Work out the finished part from the listing and answer in its coordinate system (mm). Face numbers are marked on the shaded views. Coordinates: 2 decimals unless noted, no trailing zeros. Write each loop counter-clockwise with the first axis right and the second up, starting at its lowest first coordinate (ties: lowest second). Pieces come first, ordered by that corner, then holes. Notation, with made-up numbers: M 52,4 L 71,4 A36 cw 71,39 Z; hole C 8.25,53.5 d11. An arc over 180 degrees is marked long. Use CSV: the item, a comma, the result in double quotes.
from build123d import *


with BuildPart() as part:
    # Sketch1 → Revolve1 (revolve)
    with BuildSketch(Plane.XZ):
        with BuildLine():
            Line((14.2875, 0.508), (14.2875, 5.89534))
            Line((14.2875, 5.89534), (13.97, 5.89534))
            Line((13.97, 5.89534), (13.97, 6.40334))
            Line((13.97, 6.40334), (15.4305, 6.40334))
            Line((15.4305, 6.40334), (15.5575, 6.53034))
            Line((15.5575, 6.53034), (15.5575, 7.80034))
            Line((15.5575, 7.80034), (15.4305, 7.92734))
            Line((15.4305, 7.92734), (6.35, 7.92734))
            Line((6.35, 7.92734), (6.35, 0))
            Line((6.35, 0), (13.7795, 0))
            ThreePointArc((13.7795, 0), (14.138710245, 0.148789755), (14.2875, 0.508))
        make_face()
    revolve(axis=Axis((0, 0, 7.92734), (0, 0, -1)))


solid = part.part
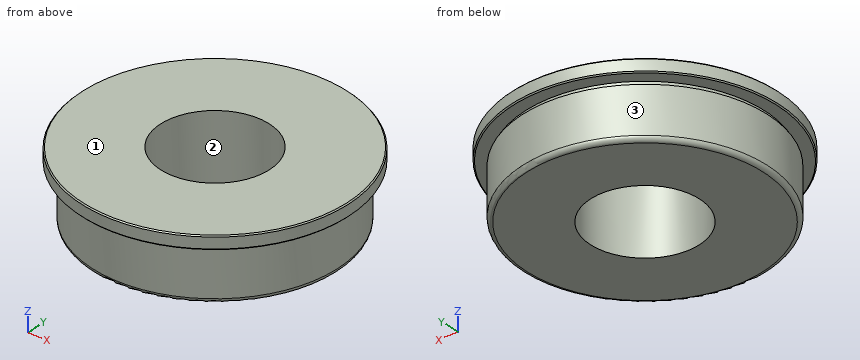
Item 1: Given pin 1 (3 mm diameter, centred on y = -10, z = 6, fed in from -X); pin 2 (2 mm diameter, centred on y = 11, z = 2.5, fed in from +X); pin 3 (1 mm diameter, centred on y = -6, z = 4, fed in from -X), each flat-ended and moving along its own axis, determine where each tip first touches the part or whether it passes through.
Answer:
pin 1,"stops at x = -12.97"
pin 2,"stops at x = 10.2"
pin 3,"stops at x = -13.19"
Item 2: The part is cut by section A-A (x = 0). Write down the section's boundary in (y, z).
Answer:
outline,"M -15.56,6.53 L -15.43,6.4 L -13.97,6.4 L -13.97,5.9 L -14.29,5.9 L -14.29,0.51 A0.51 ccw -13.78,0 L -6.35,0 L -6.35,7.93 L -15.43,7.93 L -15.56,7.8 Z; M 6.35,0 L 13.78,0 A0.51 ccw 14.29,0.51 L 14.29,5.9 L 13.97,5.9 L 13.97,6.4 L 15.43,6.4 L 15.56,6.53 L 15.56,7.8 L 15.43,7.93 L 6.35,7.93 Z"
Item 3: Consider probe 1 along X at (y, z) = (0, 4); probe 2 along Y at (x, z) = (0, 6). Determine where each line is inside the solid, lowest interval first.
Answer:
probe 1,"x = -14.29 to -6.35, 6.35 to 14.29"
probe 2,"y = -13.97 to -6.35, 6.35 to 13.97"
Item 4: For a pull along X with two mould halves and no side action, classify the marked faces 1, 2 and 3 as released by +X, released by -X, zero draft, split by the parting line, or undercut.
Answer:
face 1,"zero draft"
face 2,"undercut"
face 3,"split by the parting line"
